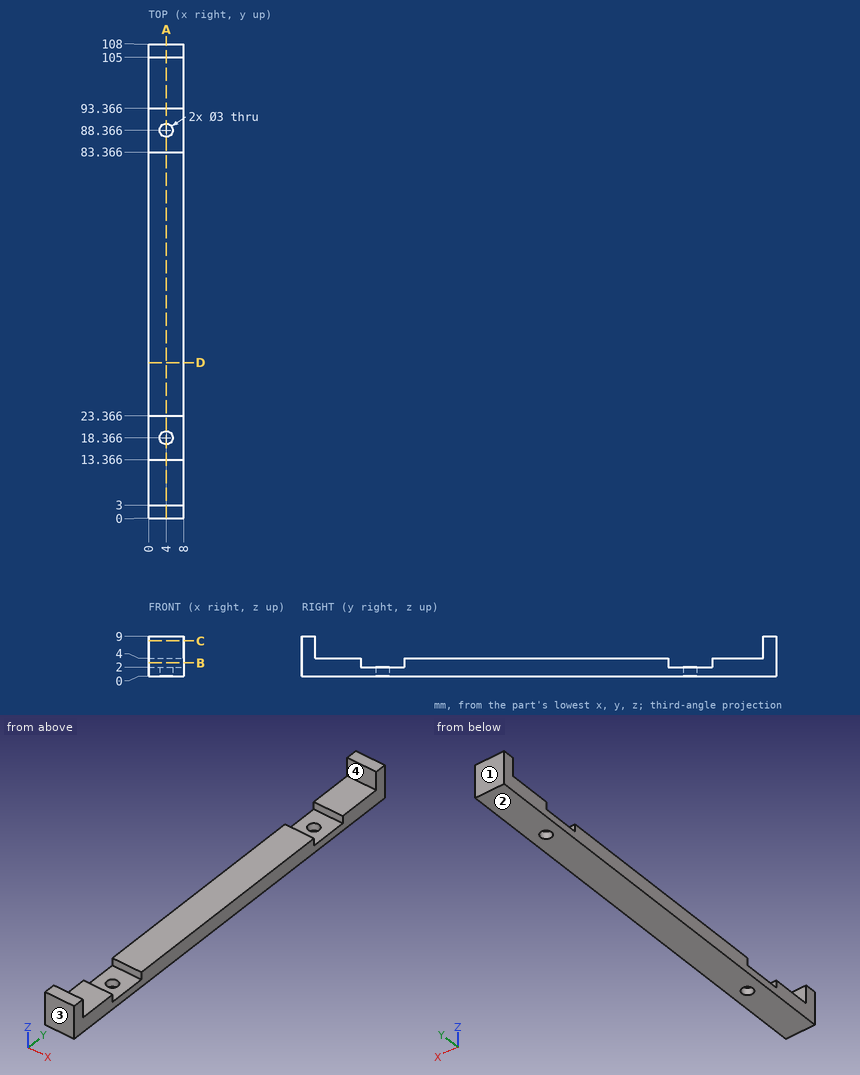
The drawing under review shows one solid part. Ordinate dimensions are in mm from its lowest x, y, z. Coordinates: 2 decimals unless noted, no trailing zeros. Write each loop counter-clockwise with the first axis right and the second up, starting at its lowest first coordinate (ties: lowest second). Pieces come first, ordered by that corner, then holes.
1) Mouldability with a two-part tool opening along Y and no side actions: class the marked faces 1, 2, 3 and 4 as +Y half, -Y half, draft (parallel to the pull), parting line (faces both ways), or undercut.
2) Insertion check: pin 1 (1 mm diameter, centred on x = 4.5, y = 47, fed in from -Z); pin 2 (2 mm diameter, centred on x = 3, y = 35.5, fed in from +Z); pin 3 (4 mm diameter, centred on x = 2, y = 16.5, fed in from +Z). Each pin has a flat end and moves straight along its axis. Give the tip position at first contact, or say it passes through.
3) Add section C-C (z = 8). Write out the cut boundary in (x, y).
4) To check wall thickness, follow L1, parallel to Y at x = 4, z = 0.6; L2, parallel to Y at x = 7, z = 8.75; L3, parallel to Z at x = 4, y = 52. State the ranges of each line that lie inside material, in increasing order.
5) Add section D-D (y = 35.5). Write out the cut boundary in (x, z), plus the area to 3 significant figures.
6) Add section A-A (x = 4). Write out the cut boundary in (y, z).
7) Add section B-B (z = 3). Write out the cut boundary in (x, y), plus the area to 3 significant figures.
Check result:
1. face 1: +Y half
1. face 2: draft
1. face 3: -Y half
1. face 4: undercut
2. pin 1: stops at z = 0
2. pin 2: stops at z = 4
2. pin 3: stops at z = 2
3. outline: (0, 0) - (8, 0) - (8, 3) - (0, 3) - close; (0, 105) - (8, 105) - (8, 108) - (0, 108) - close
4. L1: y = 0 to 16.87, 19.87 to 86.87, 89.87 to 108
4. L2: y = 0 to 3, 105 to 108
4. L3: z = 0 to 4
5. outline: (0, 0) - (8, 0) - (8, 4) - (0, 4) - close
5. area: 32.0 mm2
6. outline: (0, 0) - (16.87, 0) - (16.87, 2) - (13.37, 2) - (13.37, 4) - (3, 4) - (3, 9) - (0, 9) - close; (19.87, 0) - (86.87, 0) - (86.87, 2) - (83.37, 2) - (83.37, 4) - (23.37, 4) - (23.37, 2) - (19.87, 2) - close; (89.87, 0) - (108, 0) - (108, 9) - (105, 9) - (105, 4) - (93.37, 4) - (93.37, 2) - (89.87, 2) - close
7. outline: (0, 0) - (8, 0) - (8, 13.37) - (0, 13.37) - close; (0, 23.37) - (8, 23.37) - (8, 83.37) - (0, 83.37) - close; (0, 93.37) - (8, 93.37) - (8, 108) - (0, 108) - close
7. area: 704 mm2
